```python
from build123d import *

# Parameters (mm, degrees)
F1_DEPTH  = 12.7
F0_R      = 72.898
F0_R_2    = 65.278
F2_DEPTH  = 12.7
F4_R      = 72.898
F5_DEPTH  = 6.35
F6_DEPTH  = 12.7
F8_W      = 150.4707932472
F8_H      = 152.4543464184
F8_R      = 72.898
F9_DEPTH  = 12.7
F9_FACE_W = 150.4707932472
F9_FACE_H = 152.4543464184
F9_FACE_R = 72.898
F12_DEPTH = 6.35
F12_TAPER = -3


# Not quite as in the source:
# - the program builds the solid bodies; features that only make, move or delete a surface that nothing else refers to are left out


with BuildPart() as f1:
    # F0 (on Top) → F1 (new body)
    with BuildSketch(Plane.XY):
        with BuildLine():
            Line((44.0266140713, 43.9798835084), (44.9402432342, 44.8622841377))
            ThreePointArc((44.9402432342, 44.8622841377), (0.0822011404, 63.499946795), (-44.8239437094, 44.9784845269))
            Line((-44.8239437094, 44.9784845269), (-43.499038361, 43.6043470536))
            Line((-43.499038361, 43.6043470536), (-11.6539793168, 10.5759582539))
            ThreePointArc((-11.6539793168, 10.5759582539), (-0.7689783294, 15.718613146), (10.5660161344, 11.662994039))
            Line((10.5660161344, 11.662994039), (44.0266140713, 43.9798835084))
        make_face()
    extrude(amount=F1_DEPTH)



with BuildPart() as f1b:
    # F0 (on Top) → F1, piece 2 (new body)
    with BuildSketch(Plane.XY):
        with BuildLine():
            ThreePointArc((6.6638546501, -63.1493708694), (47.1891587684, -42.4903906164), (63.4999938049, -0.0280496613))
            Line((63.4999938049, -0.0280496613), (61.8462218281, 0))
            Line((61.8462218281, 0), (15.7179516616, 0.78238256))
            ThreePointArc((15.7179516616, 0.78238256), (12.2084926851, -9.9307015494), (2.4344132667, -15.5479824721))
            Line((2.4344132667, -15.5479824721), (6.5514407483, -61.8841783021))
            Line((6.5514407483, -61.8841783021), (6.6638546501, -63.1493708694))
        make_face()
    extrude(amount=F1_DEPTH)


with BuildPart() as f1c:
    # F0 (on Top) → F1, piece 3 (new body)
    with BuildSketch(Plane.XY):
        with BuildLine():
            Line((-60.5164809282, 8.5368217163), (-62.8717330434, 8.9103975287))
            ThreePointArc((-62.8717330434, 8.9103975287), (-54.0323144536, -33.3580424304), (-20.2050848869, -60.1997055202))
            Line((-20.2050848869, -60.1997055202), (-19.7810930248, -59.0023835005))
            Line((-19.7810930248, -59.0023835005), (-4.2528877081, -15.1518669823))
            ThreePointArc((-4.2528877081, -15.1518669823), (-12.9594991488, -8.928466202), (-15.6728541768, 1.4239974924))
            Line((-15.6728541768, 1.4239974924), (-60.5164809282, 8.5368217163))
        make_face()
    extrude(amount=F1_DEPTH)


with BuildPart() as f2:
    # F0 (on Top) → F2 (new body)
    with BuildSketch(Plane.XY):
        Circle(F0_R)
        Circle(F0_R_2, mode=Mode.SUBTRACT)
    extrude(amount=F2_DEPTH)


with BuildPart() as f1_1:
    add(f1.part)

    add(f1b.part)  # F5 merges F1b

    add(f1c.part)  # F5 merges F1c

    add(f2.part)  # F5 merges F2
    # F4 (on Top) → F5 (join)
    with BuildSketch(Plane.XY):
        Circle(F4_R)
    extrude(amount=-F5_DEPTH)

    # F0 (on Top) → F6 (join)
    with BuildSketch(Plane.XY):
        with BuildLine():
            ThreePointArc((63.4999938049, -0.0280496613), (63.4999984512, -0.014024831), (63.5, 0))
            ThreePointArc((63.5, 0), (58.6768925787, 24.2749310465), (44.9402432342, 44.8622841377))
            Line((44.9402432342, 44.8622841377), (44.0266140713, 43.9798835084))
            ThreePointArc((44.0266140713, 43.9798835084), (50.6520952134, 36.1515995564), (55.9018661031, 27.3414386269))
            ThreePointArc((55.9018661031, 27.3414386269), (60.528045967, 14.0303191282), (61.8462218281, 0))
            Line((61.8462218281, 0), (63.4999938049, -0.0280496613))
        make_face()
        with BuildLine():
            Line((44.0266140713, 43.9798835084), (44.9402432342, 44.8622841377))
            ThreePointArc((44.9402432342, 44.8622841377), (0.0822011404, 63.499946795), (-44.8239437094, 44.9784845269))
            Line((-44.8239437094, 44.9784845269), (-43.499038361, 43.6043470536))
            Line((-43.499038361, 43.6043470536), (-11.6539793168, 10.5759582539))
            ThreePointArc((-11.6539793168, 10.5759582539), (-0.7689783294, 15.718613146), (10.5660161344, 11.662994039))
            Line((10.5660161344, 11.662994039), (44.0266140713, 43.9798835084))
        make_face()
        with BuildLine():
            ThreePointArc((6.6638546501, -63.1493708694), (47.1891587684, -42.4903906164), (63.4999938049, -0.0280496613))
            Line((63.4999938049, -0.0280496613), (61.8462218281, 0))
            Line((61.8462218281, 0), (15.7179516616, 0.78238256))
            ThreePointArc((15.7179516616, 0.78238256), (12.2084926851, -9.9307015494), (2.4344132667, -15.5479824721))
            Line((2.4344132667, -15.5479824721), (6.5514407483, -61.8841783021))
            Line((6.5514407483, -61.8841783021), (6.6638546501, -63.1493708694))
        make_face()
        with BuildLine():
            Line((-43.499038361, 43.6043470536), (-44.8239437094, 44.9784845269))
            ThreePointArc((-44.8239437094, 44.9784845269), (-56.7874671273, 28.4153757192), (-62.8717330434, 8.9103975287))
            Line((-62.8717330434, 8.9103975287), (-60.5164809282, 8.5368217163))
            ThreePointArc((-60.5164809282, 8.5368217163), (-55.6398831968, 27.8331682386), (-43.499038361, 43.6043470536))
        make_face()
        with BuildLine():
            ThreePointArc((-20.2050848869, -60.1997055202), (-6.929383847, -63.1207861128), (6.6638546501, -63.1493708694))
            Line((6.6638546501, -63.1493708694), (6.5514407483, -61.8841783021))
            ThreePointArc((6.5514407483, -61.8841783021), (-6.7699416658, -61.8606562351), (-19.7810930248, -59.0023835005))
            Line((-19.7810930248, -59.0023835005), (-20.2050848869, -60.1997055202))
        make_face()
        with BuildLine():
            Line((-60.5164809282, 8.5368217163), (-62.8717330434, 8.9103975287))
            ThreePointArc((-62.8717330434, 8.9103975287), (-54.0323144536, -33.3580424304), (-20.2050848869, -60.1997055202))
            Line((-20.2050848869, -60.1997055202), (-19.7810930248, -59.0023835005))
            Line((-19.7810930248, -59.0023835005), (-4.2528877081, -15.1518669823))
            ThreePointArc((-4.2528877081, -15.1518669823), (-12.9594991488, -8.928466202), (-15.6728541768, 1.4239974924))
            Line((-15.6728541768, 1.4239974924), (-60.5164809282, 8.5368217163))
        make_face()
    extrude(amount=F6_DEPTH)



with BuildPart() as f6:
    # F0 (on Top) → F6, piece 2 (new body)
    with BuildSketch(Plane.XY):
        Circle(F0_R)
        Circle(F0_R_2, mode=Mode.SUBTRACT)
    extrude(amount=F6_DEPTH)


with BuildPart() as f1_2:
    add(f1_1.part)

    add(f6.part)  # F9 merges F6
    # F8 (on face) → F9 (join)
    with BuildSketch(Plane.XY):
        Rectangle(F8_W, F8_H)
        Circle(F8_R, mode=Mode.SUBTRACT)
    extrude(amount=F9_DEPTH)

    # F9_face (on face) → F12 (join)
    with BuildSketch(Plane(origin=(0, 0, 0), x_dir=(1, 0, 0), z_dir=(0, 0, -1))):
        Rectangle(F9_FACE_W, F9_FACE_H)
        Circle(F9_FACE_R, mode=Mode.SUBTRACT)
    extrude(amount=F12_DEPTH, taper=F12_TAPER)


solid = f1_2.part
```
Source: CAD feature listing. Evaluate the final solid. Frame: model axes, mm. A direction names the side the tool comes from. Coordinates: 2 decimals unless noted, no trailing zeros. One line per item, written item: value.
1) Mould query, pull axis Y, two halves, no side actions, for faces 5 (the face through (0, 2, -6.35)), 6 (the face through (-1, 76.227, 6)), 7 (the face through (-0.94, 15.71, 6.26)). Classes: released by +Y, released by -Y, zero draft, split by the parting line, or undercut.
Computed values:
face 5: zero draft
face 6: released by +Y
face 7: undercut
2) Ray query, line 1 (Y direction, x = 0, z = 9); line 2 (X direction, y = 58, z = 12); line 3 (Y direction, x = -26, z = 2). Return the intervals inside material, ascending. Write a range as [from, to].
Computed values:
line 1: y = [-76.23, -65.28], [-63.5, -62.23], [15.74, 63.5], [65.28, 76.23]
line 2: x = [-75.24, -29.95], [-25.85, 25.85], [29.95, 75.24]
line 3: y = [-76.23, -59.88], [-57.93, 3.06], [25.46, 57.93], [59.88, 76.23]
3) Contact query for flat-ended pins moving along their axis: pin 1 (10 mm diameter, centred on x = -33, z = 9.5, fed in from +Y); pin 2 (5 mm diameter, centred on y = 18.5, z = 0.5, fed in from +X); pin 3 (3 mm diameter, centred on x = -55.5, z = 9.5, fed in from -Y); pin 4 (10 mm diameter, centred on x = 44.5, z = -1.5, fed in from +Y). Output: stop coordinate, or through.
Computed values:
pin 1: stops at y = 76.23
pin 2: stops at x = 75.34
pin 3: stops at y = -76.23
pin 4: stops at y = 76.56
4) Reachability of faces 1 (the face through (13, -13, 12.7)), 2 (the face through (-1, -76.227, 6)), 3 (the face through (4.464, -38.392, 6.261)), 4 (the face through (-75.235, -1, 6)) from +Z, -Z, +X, -X, +Y, -Y: full face, straight path, thin tool, end or side. Return the list, or none.
Computed values:
face 1: +Z, +X, -X, +Y, -Y
face 2: +Z, +X, -X, -Y
face 3: +Z
face 4: +Z, -X, +Y, -Y
5) Cut plane A-A on z = 9.5. State how many separate pieces and enclosed holes the cut face has, plus the area to 3 significant figures.
Computed values:
separate pieces: 2
enclosed holes: 2
area: 18,100 mm^2
